from build123d import *

# Parameters (mm, degrees)
F0_R     = 1.75
F1_DEPTH = 2
F2_SIZE  = 1.2


with BuildPart() as f1:
    # F0 (on Front) → F1 (new body)
    with BuildSketch(Plane.XZ):
        with BuildLine():
            Line((40, 38), (-40, 38))
            ThreePointArc((-40, 38), (-42.828427, 36.828427), (-44, 34))
            Line((-44, 34), (-44, 4))
            ThreePointArc((-44, 4), (-42.828427, 1.171573), (-40, 0))
            Line((-40, 0), (40, 0))
            ThreePointArc((40, 0), (42.828427, 1.171573), (44, 4))
            Line((44, 4), (44, 34))
            ThreePointArc((44, 34), (42.828427, 36.828427), (40, 38))
        make_face()
        with Locations((-40.8, 5)):
            Circle(F0_R, mode=Mode.SUBTRACT)
        with Locations((40.8, 5)):
            Circle(F0_R, mode=Mode.SUBTRACT)
        with Locations((-40.8, 33)):
            Circle(F0_R, mode=Mode.SUBTRACT)
        with Locations((40.8, 33)):
            Circle(F0_R, mode=Mode.SUBTRACT)
    extrude(amount=F1_DEPTH)

    # F2
    f2_edges = [f1.edges().sort_by_distance(p)[0] for p in [
        (-42.55, -2, 33),
        (-42.55, -2, 5),
        (39.05, -2, 5),
        (39.05, -2, 33),
    ]]
    chamfer(f2_edges, length=F2_SIZE)


solid = f1.part
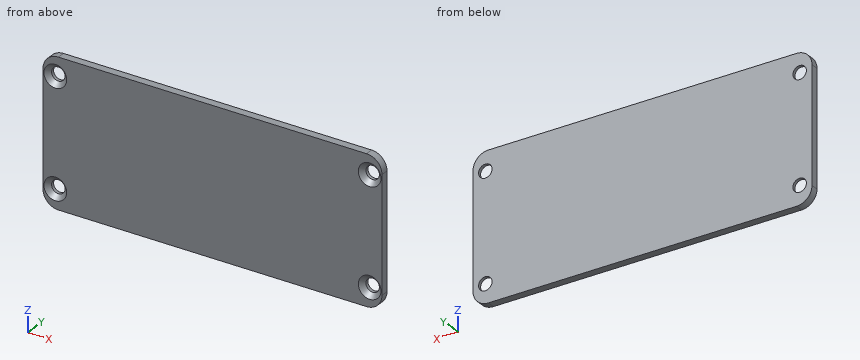
Can you work these out from the model? Positions are in its coordinate system, mm. Round coordinates to 2 decimals unless told otherwise and drop trailing zeros. Write each loop counter-clockwise with the first axis right and the second up, starting at its lowest first coordinate (ties: lowest second). Pieces come first, ordered by that corner, then holes. Notation, with made-up numbers: (81, 61.25) -> (106, 61.25) arc R24 cw to (106, 83.25) -> close; hole circle Ø9 at (67.25, 61.25). An arc over 180 degrees is marked (long way). Use one line per item in the form item = value. Start each with the question number.
Q1. If I drill on probe 1 along X at (y, z) = (-1.1, 4); probe 2 along Z at (x, y) = (40.8, -0.4); probe 3 along X at (y, z) = (-1.75, 3.5) (3 decimals), over which ranges is the centre line in solid material (lowest first)? Write a range as [from, to].
Q2. Imagine slicing it at A-A (z = 5). Please give me the cut outline in (x, y), then the cut area to 3 significant figures.
Q3. Imagine slicing it at C-C (x = 40.8). Please give me the cut outline in (y, z).
Q4. I'm going to push flat-ended pins straight in: P1, Ø5.5, axis at x = 40.8, z = 33, coming from the +Y side; P2, Ø3, axis at x = 40.8, z = 5, coming from the +Y side. Where does each tip first touch, or does it pass through?
Q5. Imagine slicing it at B-B (y = -1.5). Please give me the cut outline in (x, z).
Worked out:
q1.probe_1 = [-44, -42.59], [-39.01, 39.01], [42.59, 44]
q1.probe_2 = [0.08, 3.25], [6.75, 31.25], [34.75, 37.92]
q1.probe_3 = [-43.969, -43.045], [-38.555, 38.555], [43.045, 43.969]
q2.outline = (-44, -2) -> (-43.75, -2) -> (-42.55, -0.8) -> (-42.55, 0) -> (-44, 0) -> close; (-39.05, -0.8) -> (-37.85, -2) -> (37.85, -2) -> (39.05, -0.8) -> (39.05, 0) -> (-39.05, 0) -> close; (42.55, -0.8) -> (43.75, -2) -> (44, -2) -> (44, 0) -> (42.55, 0) -> close
q2.area = 159 mm^2
q3.outline = (-2, 0.08) -> (0, 0.08) -> (0, 3.25) -> (-0.8, 3.25) -> (-2, 2.05) -> close; (-2, 7.95) -> (-0.8, 6.75) -> (0, 6.75) -> (0, 31.25) -> (-0.8, 31.25) -> (-2, 30.05) -> close; (-2, 35.95) -> (-0.8, 34.75) -> (0, 34.75) -> (0, 37.92) -> (-2, 37.92) -> close
q4.P1 = 0
q4.P2 = through
q5.outline = (-44, 4) arc R4 ccw to (-40, 0) -> (40, 0) arc R4 ccw to (44, 4) -> (44, 34) arc R4 ccw to (40, 38) -> (-40, 38) arc R4 ccw to (-44, 34) -> close; hole circle Ø4.9 at (-40.8, 5); hole circle Ø4.9 at (-40.8, 33); hole circle Ø4.9 at (40.8, 5); hole circle Ø4.9 at (40.8, 33)
